Autodesk Inventor part; units mm, degrees
ref_plane "YZ Plane" through (0, 0, 0) normal (1, 0, 0) x (0, 1, 0)
ref_plane "XZ Plane" through (0, 0, 0) normal (0, 1, 0) x (-1, 0, 0)
ref_plane "XY Plane" through (0, 0, 0) normal (0, 0, 1) x (1, 0, 0)
sketch "Sketch1" plane through (0, 0, 0) normal (0, 1, 0) x (-1, 0, 0)
  line L0 (-8.89, -45.72) -> (8.89, -45.72)
  line L1 (8.89, -45.72) -> (8.89, 45.72)
  line L2 (8.89, 45.72) -> (-8.89, 45.72)
  line L3 (-8.89, 45.72) -> (-8.89, -45.72)
  line L4 (-8.89, -45.72) -> (8.89, 45.72) construction
  line L5 (8.89, -45.72) -> (-8.89, 45.72) construction
  point P0 (0, 0)
  dimension "d0" = 17.78
  dimension "d1" = 91.44
extrude "Plate1" add sketch "Sketch1" along normal blind 0.9144
sketch "Sketch2" plane through (8.89, 0.9144, -45.72) normal (0.6946584, -0.7193398, 0) x (0.7193398, 0.6946584, 0)
  line L0 (0, 91.44) -> (0, 0)
  line L1 (0, 0) -> (17.4106, 0)
  line L2 (17.4106, 0) -> (17.4106, 91.44)
  line L3 (17.4106, 91.44) -> (0, 91.44)
edge flange "Flange1" height 17.78 angle 44 thickness 0.9144 bend radius 0.762 thickness toward (0.6946584, -0.7193398, 0) relief tear relief width 0.9144 relief depth 0.4572 edges at (8.89, 0.9144, 0) wall of the first edge with corners at (8.89, 0.9144, 45.72) (8.89, 0.9144, -45.72) (21.4141, 13.0088, -45.72) (21.4141, 13.0088, 45.72)
bend "Bend1"
corner "Corner1"
sketch "Sketch3" plane through (0, 0.9144, 0) normal (0, 1, 0) x (1, 0, 0)
  line L0 (-14.9938, 0) -> (27.733, 0)
  line L1 (-8.89, -45.72) -> (-8.89, 45.72)
  point P0 (0, 0)
  point P1 (0, 38.1)
  point P2 (0, -38.1)
  dimension "d13" = 76.2
  dimension "d14" = 8.89
hole "Hole1" at (0, 0.9144, -38.1) at (0, 0.9144, 38.1) direction (0, -1, 0) diameter 3.2512 end through all
sketch "Sketch4" plane through (21.4141, 13.0088, -45.72) normal (-0.6946584, 0.7193398, 0) x (0, 0, 1)
  line L0 (91.44, 0) -> (0, 0)
  line L1 (45.72, -40.2779) -> (45.72, 7.2461)
  point P0 (45.72, -24.4407)
  point P1 (19.304, -7.239)
  point P2 (72.136, -7.239)
  dimension "d22" = 7.239
  dimension "d23" = 52.832
hole "Hole2" at (16.2068, 7.9802, -26.416) at (16.2068, 7.9802, 26.416) direction (0.6946584, -0.7193398, 0) diameter 3.2512 end through all
fillet "Corner Round1" radius 6.35 4 edges at (-8.89, 0.4572, 45.72) (21.7317, 12.6799, -45.72) (-8.89, 0.4572, -45.72) (21.7317, 12.6799, 45.72)
equation "\"d20\" = Thickness"
equation "\"d29\" = Thickness"
equation "\"d2\" = Thickness"
equation "\"d3\" = BendReliefWidth"
equation "\"d4\" = BendReliefDepth"
equation "\"d5\" = MinimumRemnant"
equation "\"d6\" = TransitionRadius"
equation "\"d9\" = BendRadius"
equation "\"d10\" = CornerReliefSize"
equation "\"d11\" = GapSize"
equation "\"d12\" = JacobiRadiusSize"
equation "\"BendReliefWidth\" = Thickness"
equation "\"BendReliefDepth\" = 0.5 * Thickness"
equation "\"CornerReliefSize\" = 4 * Thickness"
equation "\"MinimumRemnant\" = 2 * Thickness"
equation "\"TransitionRadius\" = BendRadius"
equation "\"JacobiRadiusSize\" = BendRadius"
equation "\"GapSize\" = Thickness"
properties part number "J009600" material "STAINLESS STEEL, 316"
Build history of the part. All positions in model axes, mm. Coordinates: 2 decimals unless noted, no trailing zeros. Write each loop counter-clockwise with the first axis right and the second up, starting at its lowest first coordinate (ties: lowest second). Pieces come first, ordered by that corner, then holes. Notation, with made-up numbers: (-4.5, 13.25) -> (3.5, 13.25) arc R19 cw to (3.5, 35.25) -> close; hole circle Ø7 at (57.5, 5). An arc over 180 degrees is marked (long way). Use CSV: the item, a comma, the result in double quotes. Start each with the question number.
Q1. Cut at B-B, the plane x = 0. List the corners of the cut face in (y, z).
Q2. Cut at C-C, the plane z = -0.5. List the corners of the cut face in (x, y), then the cut area to 3 significant figures.
Q3. Drill centre lines: probe 1 along Z at (x, y) = (0, 0.3); probe 2 along Y at (x, z) = (-2.5, -8); probe 3 along X at (y, z) = (0.4, -38.1). Where is each one in solid material? Low to high.
Q4. Cut at D-D, the plane z = -37.5. List the corners of the cut face in (x, y).
Q5. Flat gauge pins, fed straight in: pin 1 Ø5 at (x, z) = (0, -38.1) entering from +Y; pin 2 Ø2 at (y, z) = (6, 26) entering from -X; pin 3 Ø4 at (x, y) = (5, 3.5) entering from -Z; pin 4 Ø4 at (x, z) = (7, 16) entering from +Y. Where does each tip first touch, or does it go through?
Q6. Pull direction Z, two halves, no side cores. Call faces 1 (the cylindrical face through (20.36, 11.35, -43.91)), 2 (the cylindrical face through (-7.08, 0.46, 43.81)), 3 (the flat face through (0, 0.914, 1)), 4 (the cylindrical face through (16.977, 8.079, -24.914)): released by +Z, released by -Z, zero draft, split by the parting line, or undercut.
Q7. Cut at A-A, the plane z = 38.1. List the corners of the cut face in (x, y).
Checked values:
1,outline,"(0, -45.72) -> (0.91, -45.72) -> (0.91, -39.73) -> (0, -39.73) -> close; (0, -36.47) -> (0.91, -36.47) -> (0.91, 36.47) -> (0, 36.47) -> close; (0, 39.73) -> (0.91, 39.73) -> (0.91, 45.72) -> (0, 45.72) -> close"
2,outline,"(-8.89, 0) -> (8.58, 0) arc R1.68 ccw to (9.75, 0.47) -> (22.05, 12.35) -> (21.41, 13.01) -> (9.11, 1.13) arc R0.76 cw to (8.58, 0.91) -> (-8.89, 0.91) -> close"
2,area,"32.5 mm²"
3,probe 1,"z = -45.72 to -39.73, -36.47 to 36.47, 39.73 to 45.72"
3,probe 2,"y = 0 to 0.91"
3,probe 3,"x = -8.89 to -1.63, 1.63 to 9.67"
4,outline,"(-8.89, 0) -> (-1.51, 0) -> (-1.51, 0.91) -> (-8.89, 0.91) -> close; (1.51, 0) -> (8.58, 0) arc R1.68 ccw to (9.75, 0.47) -> (22.05, 12.35) -> (21.41, 13.01) -> (9.11, 1.13) arc R0.76 cw to (8.58, 0.91) -> (1.51, 0.91) -> close"
5,pin 1,"stops at y = 0.91"
5,pin 2,"stops at x = 13.12"
5,pin 3,"passes through"
5,pin 4,"stops at y = 1.04"
6,face 1,"released by -Z"
6,face 2,"released by +Z"
6,face 3,"zero draft"
6,face 4,"undercut"
7,outline,"(-8.89, 0) -> (-1.63, 0) -> (-1.63, 0.91) -> (-8.89, 0.91) -> close; (1.63, 0) -> (8.58, 0) arc R1.68 ccw to (9.75, 0.47) -> (22.05, 12.35) -> (21.41, 13.01) -> (9.11, 1.13) arc R0.76 cw to (8.58, 0.91) -> (1.63, 0.91) -> close"
